Geometry check sheet. Reference: the model listing, model coordinates, mm. Round coordinates to 2 decimals unless told otherwise and drop trailing zeros. Loops run counter-clockwise (first coordinate to the right, second up) from the corner with the lowest first, then second, coordinate; pieces in that order, holes last. Notation, with made-up numbers: (76.25, 9) -> (82.25, 9) arc R11 ccw to (82.25, 21) -> close; hole circle Ø6 at (64, 43.25). An arc over 180 degrees is marked (long way). Use a Markdown table: item, result. Add a question column.
Q1. Gauge pin test, flat end, axial feed: P1, Ø5, axis at y = 36.5, z = -4, coming from the -X side. Record the tip position at first contact, or that the pin passes through.
Q2. Sectioned sample at A-A, the plane y = 225. Enter the section's corners in (x, z).
Q3. Sectioned sample at B-B, the plane x = 80. Enter the section's corners in (y, z), then the cut area to 3 significant figures.
Q4. Sectioned sample at D-D, the plane y = 320. Enter the section's corners in (x, z).
Q5. Material ranges on L1, parallel to Y at x = 80, z = -7; L2, parallel to Y at x = 88.5, z = -2.25, recorded low to high.
Q6. Sectioned sample at C-C, the plane z = -5.25. Enter the section's corners in (x, y).
```python
from build123d import *

# Parameters (mm, degrees)
SKETCH1_W           = 100
SKETCH1_H           = 15
BOSS_EXTRUDE1_DEPTH = 350
SKETCH2_R           = 12.5
CUT_EXTRUDE1_DEPTH  = 16
SKETCH3_R           = 10.318452201
SKETCH3_R_2         = 11.907148997
CUT_EXTRUDE2_DEPTH  = 16


with BuildPart() as part:
    # Sketch1 → Boss-Extrude1 (new body)
    with BuildSketch(Plane(origin=(0, 0, 0), x_dir=(1, 0, 0), z_dir=(0, 1, 0))):
        with Locations((50, 7.5)):
            Rectangle(SKETCH1_W, SKETCH1_H)
    extrude(amount=BOSS_EXTRUDE1_DEPTH)

    # Sketch2 → Cut-Extrude1 (cut, through all)
    with BuildSketch(Plane.XY):
        with Locations((80, 225)):
            Circle(SKETCH2_R)
    extrude(amount=-CUT_EXTRUDE1_DEPTH, mode=Mode.SUBTRACT)

    # Sketch3 → Cut-Extrude2 (cut, through all)
    with BuildSketch(Plane.XY):
        with Locations((80, 320)):
            Circle(SKETCH3_R)
        with Locations((80, 130)):
            Circle(SKETCH3_R_2)
    extrude(amount=-CUT_EXTRUDE2_DEPTH, mode=Mode.SUBTRACT)


solid = part.part
```
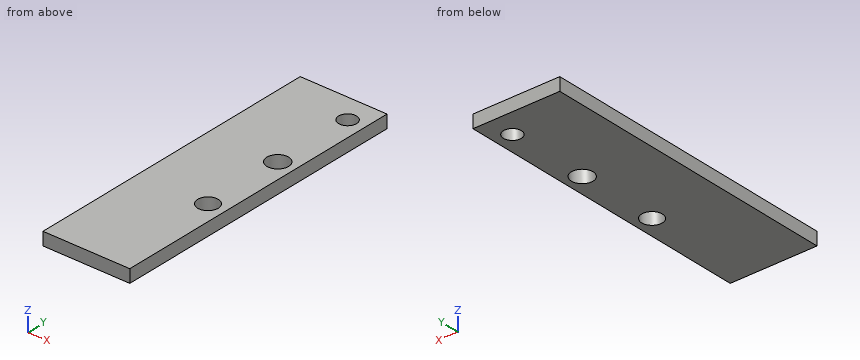
Values:
| question | item | result |
|---|---|---|
| 1 | P1 | x = 0 |
| 2 | outline | (0, -15) -> (67.5, -15) -> (67.5, 0) -> (0, 0) -> close; (92.5, -15) -> (100, -15) -> (100, 0) -> (92.5, 0) -> close |
| 3 | outline | (0, -15) -> (118.09, -15) -> (118.09, 0) -> (0, 0) -> close; (141.91, -15) -> (212.5, -15) -> (212.5, 0) -> (141.91, 0) -> close; (237.5, -15) -> (309.68, -15) -> (309.68, 0) -> (237.5, 0) -> close; (330.32, -15) -> (350, -15) -> (350, 0) -> (330.32, 0) -> close |
| 3 | area | 4,210 mm^2 |
| 4 | outline | (0, -15) -> (69.68, -15) -> (69.68, 0) -> (0, 0) -> close; (90.32, -15) -> (100, -15) -> (100, 0) -> (90.32, 0) -> close |
| 5 | L1 | 0 to 118.09, 141.91 to 212.5, 237.5 to 309.68, 330.32 to 350 |
| 5 | L2 | 0 to 121.66, 138.34 to 215.83, 234.17 to 314.15, 325.85 to 350 |
| 6 | outline | (0, 0) -> (100, 0) -> (100, 350) -> (0, 350) -> close; hole circle Ø25 at (80, 225); hole circle Ø23.81 at (80, 130); hole circle Ø20.64 at (80, 320) |
